from build123d import *

# Parameters (mm, degrees)
CYLINDER003_R     = 4
CYLINDER003_DEPTH = 12.7
CYLINDER002_R     = 4
CYLINDER002_DEPTH = 12.7
CYLINDER_R        = 4
CYLINDER_DEPTH    = 12.7
CYLINDER001_R     = 4
CYLINDER001_DEPTH = 12.7
BOX001_W          = 10.3
BOX001_H          = 10.3
BOX001_DEPTH      = 200
BOX_W             = 12.7
BOX_H             = 12.7
BOX_DEPTH         = 200


with BuildPart() as cilindro003:
    # Cylinder003 → Cylinder003 (new body)
    with BuildSketch(Plane(origin=(0, 6.35, 170), x_dir=(0, 0, -1), z_dir=(1, 0, 0))):
        Circle(CYLINDER003_R)
    extrude(amount=CYLINDER003_DEPTH)


with BuildPart() as cilindro002:
    # Cylinder002 → Cylinder002 (new body)
    with BuildSketch(Plane(origin=(0, 6.35, 30), x_dir=(0, 0, -1), z_dir=(1, 0, 0))):
        Circle(CYLINDER002_R)
    extrude(amount=CYLINDER002_DEPTH)


with BuildPart() as cilindro:
    # Cylinder → Cylinder (new body)
    with BuildSketch(Plane(origin=(6.35, 0, 15), x_dir=(1, 0, 0), z_dir=(0, 1, 0))):
        Circle(CYLINDER_R)
    extrude(amount=CYLINDER_DEPTH)


with BuildPart() as cilindro001:
    # Cylinder001 → Cylinder001 (new body)
    with BuildSketch(Plane(origin=(6.35, 0, 185), x_dir=(1, 0, 0), z_dir=(0, 1, 0))):
        Circle(CYLINDER001_R)
    extrude(amount=CYLINDER001_DEPTH)


with BuildPart() as obj1:
    # Box001 → Box001 (new body)
    with BuildSketch(Plane(origin=(1.2, 1.2, 0), x_dir=(1, 0, 0), z_dir=(0, 0, 1))):
        with Locations((5.15, 5.15)):
            Rectangle(BOX001_W, BOX001_H)
    extrude(amount=BOX001_DEPTH)


with BuildPart() as obj2:
    # Box → Box (new body)
    with BuildSketch(Plane.XY):
        with Locations((6.35, 6.35)):
            Rectangle(BOX_W, BOX_H)
    extrude(amount=BOX_DEPTH)

    # Cut: cut obj1
    add(obj1.part, mode=Mode.SUBTRACT)

    # Cut001: cut Cilindro001
    add(cilindro001.part, mode=Mode.SUBTRACT)

    # Cut002: cut Cilindro
    add(cilindro.part, mode=Mode.SUBTRACT)

    # Cut003: cut Cilindro002
    add(cilindro002.part, mode=Mode.SUBTRACT)

    # Cut004: cut Cilindro003
    add(cilindro003.part, mode=Mode.SUBTRACT)


solid = obj2.part
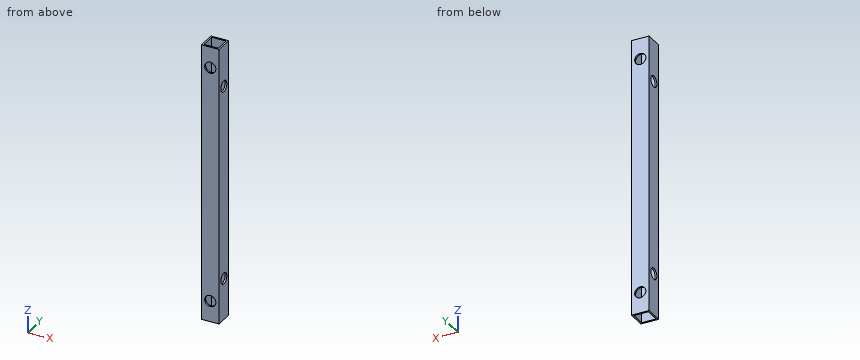
Design review of the part built by this model. Coordinates are the model's own, in mm. Round coordinates to 2 decimals unless told otherwise and drop trailing zeros. Write each loop counter-clockwise with the first axis right and the second up, starting at its lowest first coordinate (ties: lowest second). Pieces come first, ordered by that corner, then holes. Notation, with made-up numbers: (54, -12) - (93, -12) arc R29 cw to (93, 23) - close; hole circle Ø10 at (77, 83). An arc over 180 degrees is marked (long way). Return JSON: item names as keys, results as strings. Group by question number.
Item 1: We need section C-C on z = 170. Write out the cut boundary in (x, y), and give its area (3 significant figures).
Item 2: We need section A-A on y = 6.35. Write out the cut boundary in (x, z), and give its area (3 significant figures).
Item 3: For probe 1 along Z at (x, y) = (0.45, 6.35); probe 2 along Y at (x, z) = (4.5, 175.5), list the stretches that pass through material, from the lowest coordinate up. Write a range as [from, to].
Item 4: We need section B-B on x = 6.35. Write out the cut boundary in (y, z), and give its area (3 significant figures).
Item 5: We need section D-D on z = 48. Write out the cut boundary in (x, y).
Model answer:
{
 "1": {"outline": "(0, 0) - (12.7, 0) - (12.7, 2.35) - (11.5, 2.35) - (11.5, 1.2) - (1.2, 1.2) - (1.2, 2.35) - (0, 2.35) - close; (0, 10.35) - (1.2, 10.35) - (1.2, 11.5) - (11.5, 11.5) - (11.5, 10.35) - (12.7, 10.35) - (12.7, 12.7) - (0, 12.7) - close", "area": "36.0 mm²"},
 "2": {"outline": "(0, 0) - (1.2, 0) - (1.2, 26) - (0, 26) - close; (0, 34) - (1.2, 34) - (1.2, 166) - (0, 166) - close; (0, 174) - (1.2, 174) - (1.2, 200) - (0, 200) - close; (11.5, 0) - (12.7, 0) - (12.7, 26) - (11.5, 26) - close; (11.5, 34) - (12.7, 34) - (12.7, 166) - (11.5, 166) - close; (11.5, 174) - (12.7, 174) - (12.7, 200) - (11.5, 200) - close", "area": "442 mm²"},
 "3": {"probe 1": "z = [0, 26], [34, 166], [174, 200]", "probe 2": "y = [0, 1.2], [11.5, 12.7]"},
 "4": {"outline": "(0, 0) - (1.2, 0) - (1.2, 11) - (0, 11) - close; (0, 19) - (1.2, 19) - (1.2, 181) - (0, 181) - close; (0, 189) - (1.2, 189) - (1.2, 200) - (0, 200) - close; (11.5, 0) - (12.7, 0) - (12.7, 11) - (11.5, 11) - close; (11.5, 19) - (12.7, 19) - (12.7, 181) - (11.5, 181) - close; (11.5, 189) - (12.7, 189) - (12.7, 200) - (11.5, 200) - close", "area": "442 mm²"},
 "5": {"outline": "(0, 0) - (12.7, 0) - (12.7, 12.7) - (0, 12.7) - close; hole (1.2, 1.2) - (11.5, 1.2) - (11.5, 11.5) - (1.2, 11.5) - close"}
}
